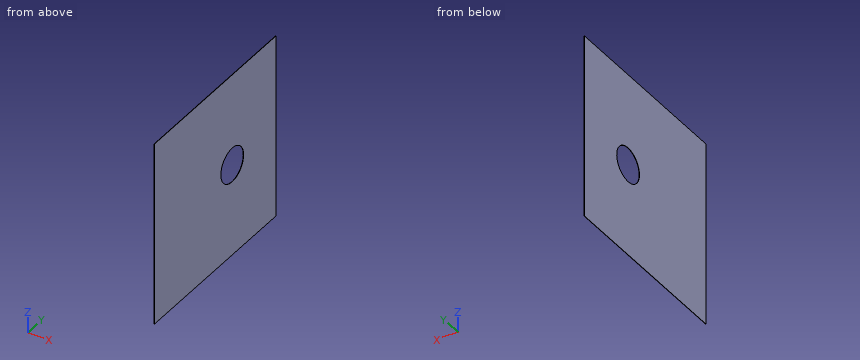
Autodesk Inventor part; units mm, degrees
ref_plane "YZ Plane" through (0, 0, 0) normal (1, 0, 0) x (0, 1, 0)
ref_plane "XZ Plane" through (0, 0, 0) normal (0, 1, 0) x (-1, 0, 0)
ref_plane "XY Plane" through (0, 0, 0) normal (0, 0, 1) x (1, 0, 0)
sketch "Sketch1" plane through (0, 0, 0) normal (1, 0, 0) x (0, 1, 0)
  line L0 (-304.8, 304.8) -> (304.8, 304.8)
  line L1 (304.8, 304.8) -> (304.8, -304.8)
  line L2 (304.8, -304.8) -> (-304.8, -304.8)
  line L3 (-304.8, -304.8) -> (-304.8, 304.8)
  line L4 (-304.8, 304.8) -> (304.8, -304.8) construction
  line L5 (304.8, 304.8) -> (-304.8, -304.8) construction
  point P0 (0, 0)
  dimension "d0" = 609.6
  dimension "d1" = 609.6
extrude "Extrusion1" add sketch "Sketch1" along normal blind 1.0668
sketch "Sketch2" plane through (1.0668, 0, 0) normal (1, 0, 0) x (0, 0, -1)
  circle A0 centre (0, 85.725) radius 57.15
  line L0 (-304.8, -304.8) -> (304.8, -304.8)
  dimension "d4" = 114.3
  dimension "d7" = 390.525
extrude "Extrusion2" cut sketch "Sketch2" against normal through all
properties part number "2221A_Copper Box Side_Hole_V1" material "Copper"
The listing builds one solid part. Answer for the finished solid, in the listing's coordinates (mm). Give positions to 0.01 mm unless a question says otherwise; leave off trailing zeros. Loops run counter-clockwise (first coordinate to the right, second up) from the corner with the lowest first, then second, coordinate; pieces in that order, holes last. Notation, with made-up numbers: (-31, 54) - (-9, 54) arc R29 ccw to (-9, 77) - close; hole circle Ø6 at (87.25, 42). An arc over 180 degrees is marked (long way). Answer as CSV lines item,"result". Start each with the question number.
Item 1: A cutting plane is placed at A-A on z = 0. Determine the outline of the cut face in (x, y) (3 decimals).
Item 2: Find the intervals of material crossed by line 1 (Y direction, x = 0.65, z = 0) (3 decimals); line 2 (Y direction, x = 0.85, z = -2.5), in increasing order. Write a range as from..to.
Item 3: A cutting plane is placed at B-B on x = 0.2. Determine the outline of the cut face in (y, z) (3 decimals), then the cut area to 3 significant figures.
Found:
1,outline,"(0, -304.8) - (1.067, -304.8) - (1.067, 28.575) - (0, 28.575) - close; (0, 142.875) - (1.067, 142.875) - (1.067, 304.8) - (0, 304.8) - close"
2,line 1,"y = -304.8..28.575, 142.875..304.8"
2,line 2,"y = -304.8..28.63, 142.82..304.8"
3,outline,"(-304.8, -304.8) - (304.8, -304.8) - (304.8, 304.8) - (-304.8, 304.8) - close; hole circle Ø114.3 at (85.725, 0)"
3,area,"361,000 mm^2"
